Verification items for the finished model (mm, model axes). A direction names the side the tool comes from. Round coordinates to 2 decimals unless told otherwise and drop trailing zeros. Write each loop counter-clockwise with the first axis right and the second up, starting at its lowest first coordinate (ties: lowest second). Pieces come first, ordered by that corner, then holes. Notation, with made-up numbers: (33, 79) - (40, 79) arc R29 cw to (40, 104) - close; hole circle Ø2 at (11, 2.5). An arc over 180 degrees is marked (long way). Answer as a JSON object with one key per item and string values.
```python
from build123d import *

# Parameters (mm, degrees)
SKETCH4_W           = 30
SKETCH4_H           = 250
BOSS_EXTRUDE3_DEPTH = 5
SKETCH5_W           = 85
SKETCH5_H           = 5
BOSS_EXTRUDE4_DEPTH = 10
SKETCH6_W           = 5
SKETCH6_H           = 240
BOSS_EXTRUDE5_DEPTH = 10
SKETCH7_W           = 8.5
SKETCH7_H           = 9
BOSS_EXTRUDE6_DEPTH = 2
FILLET2_R           = 5
FILLET3_R           = 5
SKETCH8_R           = 2.1
CUT_EXTRUDE1_DEPTH  = 432
SKETCH9_R           = 3.6
CUT_EXTRUDE2_DEPTH  = 4


# Some blends are built 0.0001 mm under size
with BuildPart() as part:
    # Sketch4 → Boss-Extrude3 (new, symmetric)
    with BuildSketch(Plane.XY):
        Polygon((-15, 125), (15, 125), (100, 125), (100, 155), (-15, 155), align=None)
        Rectangle(SKETCH4_W, SKETCH4_H)
    extrude(amount=BOSS_EXTRUDE3_DEPTH, both=True)

    # Sketch5 → Boss-Extrude4 (add)
    with BuildSketch(Plane(origin=(15, 125, -5), x_dir=(1, 0, 0), z_dir=(0, -1, 0))):
        with Locations((42.5, 2.5)):
            Rectangle(SKETCH5_W, SKETCH5_H)
    extrude(amount=BOSS_EXTRUDE4_DEPTH)

    # Sketch6 → Boss-Extrude5 (add)
    with BuildSketch(Plane(origin=(15, 0, 0), x_dir=(0, 0, -1), z_dir=(1, 0, 0))):
        with Locations((2.5, -5)):
            Rectangle(SKETCH6_W, SKETCH6_H)
    extrude(amount=BOSS_EXTRUDE5_DEPTH)

    # Sketch7 → Boss-Extrude6 (add)
    with BuildSketch(Plane.XY):
        with Locations((20.75, 110.5)):
            Rectangle(SKETCH7_W, SKETCH7_H)
    extrude(amount=BOSS_EXTRUDE6_DEPTH)

    # Fillet2
    # the kernel refuses this fillet: 5 mm, written as the material it takes off along each edge
    with BuildSketch(Plane(origin=(16.5, 125, 2), x_dir=(0, 0, -1), z_dir=(0, -1, 0))) as fillet2_piece_1:
        with BuildLine():
            CenterArc((5, 4), FILLET2_R, 180, 53.130102354)
            Line((0, 4), (0, 0))
            Line((0, 0), (2, 0))
        make_face()
    extrude(amount=29, mode=Mode.SUBTRACT)
    with BuildSketch(Plane(origin=(35, 115, 2), x_dir=(0, 0, -1), z_dir=(-1, 0, 0)), Plane(origin=(16.5, 106, 2), x_dir=(0, 0, -1), z_dir=(1, 0, 0))) as fillet2_piece_2:
        with BuildLine():
            CenterArc((5, 4), FILLET2_R, 180, 53.130102354)
            Line((0, 4), (0, 0))
            Line((0, 0), (2, 0))
        make_face()
    extrude(amount=18.5, mode=Mode.SUBTRACT)

    # Fillet3
    fillet3_edges = [part.edges().sort_by_distance(p)[0] for p in [
        (15, -125, 2.5),
        (20, -125, 0),
    ]]
    fillet(fillet3_edges, radius=FILLET3_R - 0.0001)  # a hair under: the kernel refuses the full size

    # Sketch8 → Cut-Extrude1 (cut)
    with BuildSketch(Plane(origin=(0, 0, -5), x_dir=(-1, 0, 0), z_dir=(0, 0, -1))):
        with Locations((5, -100)):
            Circle(SKETCH8_R)
        with Locations((5, 105)):
            Circle(SKETCH8_R)
        with Locations((-75, 145)):
            Circle(SKETCH8_R)
    extrude(amount=-CUT_EXTRUDE1_DEPTH, mode=Mode.SUBTRACT)

    # Sketch9 → Cut-Extrude2 (cut)
    with BuildSketch(Plane(origin=(0, 0, -5), x_dir=(-1, 0, 0), z_dir=(0, 0, -1))):
        with Locations((-75, 145)):
            Circle(SKETCH9_R)
        with Locations((5, 105)):
            Circle(SKETCH9_R)
        with Locations((5, -100)):
            Circle(SKETCH9_R)
    extrude(amount=-CUT_EXTRUDE2_DEPTH, mode=Mode.SUBTRACT)


solid = part.part
```
1. Cross-section at B-B (y = -35.5). Record the boundary of the cut face in (x, z), plus the area to 3 significant figures.
Completed:
{"outline": "(-15, -5) - (25, -5) - (25, 0) - (15, 0) - (15, 5) - (-15, 5) - close", "area": "350 mm^2"}
2. Access from +Z, -Z, +X, -X, +Y, -Y to the whole of each face (thin tool, end or side, straight path). Record for faces 4 (the face through (13, -124, 1)), 5 (the face through (16, 44, -5)), 6 (the face through (62, 115, -2)), 7 (the face through (73, 143, -1)).
Completed:
{"face 4": "+Z, +X, -Y", "face 5": "-Z, +X, -X, +Y, -Y", "face 6": "+Z, -Z, +X, -Y", "face 7": "-Z"}
3. Cross-section at A-A (x = 48.5). Record the boundary of the cut face in (y, z), plus the area to 3 significant figures.
Completed:
{"outline": "(115, -5) - (155, -5) - (155, 5) - (125, 5) - (125, 0) - (115, 0) - close", "area": "350 mm^2"}
4. Material ranges on probe 1 along Y at (x, z) = (-5, 2.9); probe 2 along X at (y, z) = (145, -2.3); probe 3 along Y at (x, z) = (75, 3.4), recorded low to high. Write a range as from..to.
Completed:
{"probe 1": "y = -125..-102.1, -97.9..102.9, 107.1..155", "probe 2": "x = -15..71.4, 78.6..100", "probe 3": "y = 125..142.9, 147.1..155"}
5. Mould release check, pull along Y, two halves, no side actions. Record for faces 1 (the face through (73.065, 148.036, -3.028)), 2 (the face through (100, 135, 0)), 3 (the face through (19, -123, -1)): released by +Y, released by -Y, zero draft, split by the parting line, or undercut.
Completed:
{"face 1": "undercut", "face 2": "zero draft", "face 3": "released by -Y"}
6. Go/stop test with flat-tipped pins: pin 1 (2 mm diameter, centred on x = 74.5, y = 145.5, fed in from -Z); pin 2 (2 mm diameter, centred on y = 49.5, z = -0.5, fed in from +X); pin 3 (4 mm diameter, centred on x = 43, z = 3.5, fed in from -Y); pin 4 (6 mm diameter, centred on x = -5, y = 105, fed in from -Z). Record where each tip stops, or that it passes through.
Completed:
{"pin 1": "passes through", "pin 2": "stops at x = 25", "pin 3": "stops at y = 125", "pin 4": "stops at z = -1"}
